Autodesk Inventor part; units mm, degrees
ref_plane "YZ Plane" through (0, 0, 0) normal (1, 0, 0) x (0, 1, 0)
ref_plane "XZ Plane" through (0, 0, 0) normal (0, 1, 0) x (-1, 0, 0)
ref_plane "XY Plane" through (0, 0, 0) normal (0, 0, 1) x (1, 0, 0)
sketch "Sketch1" plane through (0, 0, 0) normal (0, 1, 0) x (-1, 0, 0)
  line L0 (0, 0) -> (9.5, 0)
  line L1 (9.5, 0) -> (9.5, -39)
  line L2 (9.5, -39) -> (0, -39)
  line L3 (0, -39) -> (0, 0)
  dimension "d0" = 9.5
  dimension "d2" = 39
extrude "Extrusion1" add sketch "Sketch1" along normal blind 65
sketch "Sketch2" plane through (0, 0, 0) normal (1, 0, 0) x (0, 0, -1)
  line L0 (39, 65) -> (0, 65)
  line L1 (0, 65) -> (39, 0)
  circle A0 centre (19.5, 32.5) radius 2.65
  point P0 (0, 0)
  dimension "d5" = 5.3
extrude "Extrusion2" cut sketch "Sketch2" against normal through all
properties part number "TENSOR"
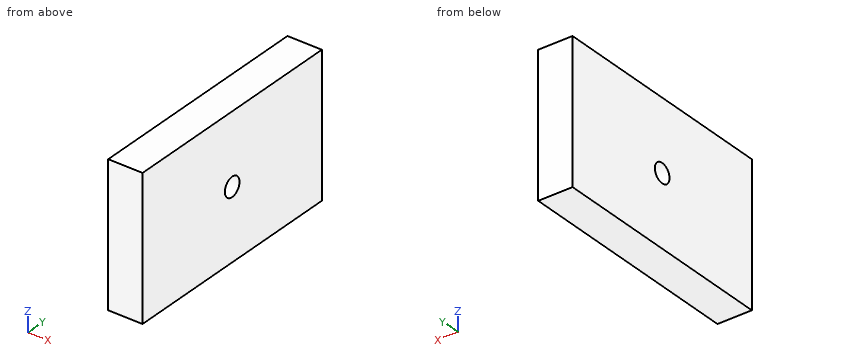
Work out the finished part from the listing and answer in its coordinate system (mm). Give positions to 0.01 mm unless a question says otherwise; leave off trailing zeros. Loops run counter-clockwise (first coordinate to the right, second up) from the corner with the lowest first, then second, coordinate; pieces in that order, holes last. Notation, with made-up numbers: (-31.5, 73.25) -> (-3.5, 73.25) arc R8 ccw to (-3.5, 87.25) -> close; hole circle Ø11 at (33.5, -32). An arc over 180 degrees is marked (long way). Use a Markdown table: item, result. Add a question column.
1. Find the intervals of material crossed by probe 1 along Y at (x, z) = (-5.75, -19.5); probe 2 along Z at (x, y) = (-5, 32.5); probe 3 along Y at (x, z) = (-3.75, -20.5), in increasing order.
2. A flat-ended cylindrical pin translates along its axis: pin 1 Ø4 at (y, z) = (32.5, -19.5) entering from -X. Find the tip coordinate at first contact, or state that the pin passes through.
3. Section A-A on z = -19.5 is taken. Determine the outline of the cut face in (x, y).
4. Section B-B on y = 32.5 is taken. Determine the outline of the cut face in (x, z).
Results below:
| question | item | result |
|---|---|---|
| 1 | probe 1 | y = 0 to 29.85, 35.15 to 65 |
| 1 | probe 2 | z = -39 to -22.15, -16.85 to 0 |
| 1 | probe 3 | y = 0 to 30.05, 34.95 to 65 |
| 2 | pin 1 | passes through |
| 3 | outline | (-9.5, 0) -> (0, 0) -> (0, 29.85) -> (-9.5, 29.85) -> close; (-9.5, 35.15) -> (0, 35.15) -> (0, 65) -> (-9.5, 65) -> close |
| 4 | outline | (-9.5, -39) -> (0, -39) -> (0, -22.15) -> (-9.5, -22.15) -> close; (-9.5, -16.85) -> (0, -16.85) -> (0, 0) -> (-9.5, 0) -> close |
